Design review of the part built by this model. Coordinates are the model's own, in mm. A direction names the side the tool comes from. Coordinates: 2 decimals unless noted, no trailing zeros. Loops run counter-clockwise (first coordinate to the right, second up) from the corner with the lowest first, then second, coordinate; pieces in that order, holes last. Notation, with made-up numbers: (65, 1.5) -> (114, 1.5) arc R20 cw to (114, 27.5) -> close; hole circle Ø3 at (87.5, -12.75). An arc over 180 degrees is marked (long way). Use a Markdown table: item, result. Add a question column.
Q1. Take a section at B-B on x = -6.5. Write out the cut boundary in (y, z), plus the area to 3 significant figures.
Q2. For faces 4 (the face through (3, 1, -7)), 5 (the face through (-7, 5, -9)), 6 (the face through (-3.9, 5.1, 9.5)), list the 3-axis set-ups (+Z, -Z, +X, -X, +Y, -Y) from which the entire face can be reached by the end or side of a thin tool; tool diameter is ignored.
Q3. Take a section at D-D on y = 5. Count the separate pieces of the cut face and the enclosed holes in it, plus the area to 3 significant figures.
Q4. Take a section at C-C on z = -8. Write out the cut boundary in (x, y).
Q5. Clearance check with flat-ended pins moving along their axes: pin 1 Ø0.5 at (y, z) = (1, 7.5) entering from +X; pin 2 Ø5 at (y, z) = (2, 0.5) entering from +X; pin 3 Ø1.4 at (x, z) = (-13, 8.5) entering from -Y. State where each tip first meets the part, or that it passes through.
Q6. Take a section at A-A on z = 4. Write out the cut boundary in (x, y), plus the area to 3 significant figures.
Q7. For probe 1 along Z at (x, y) = (-4, 7.5); probe 2 along Z at (x, y) = (-11, 7.25); probe 3 along Y at (x, z) = (-3.5, -4.25), list the stretches that pass through material, from the lowest coordinate up.
Q8. Draft analysis for pull direction Y (two halves, no side actions). For faces 1 (the face through (5.15, 5.08, -9.51)), 2 (the face through (-9, 5, 10)), 3 (the face through (-12, 2, -8)), state which applies: pulls with the +Y half, pulls with the -Y half, needs draft (parallel to the pull), parting line crosses it, or undercut.
from build123d import *

# Parameters (mm, degrees)
BASE_DEPTH          = 1.6
SKETCH4_R           = 1.85
ONESIDE_DEPTH       = 1
ANOTHERSIDE_DEPTH   = 1.3
SKETCH5_3_R         = 1.85
PIN_DEPTH           = 1
BOSS_EXTRUDE9_DEPTH = 1.2


with BuildPart() as part:
    # Sketch3 → Base (new body)
    with BuildSketch(Plane(origin=(0, 0, 0), x_dir=(1, 0, 0), z_dir=(0, 1, 0))):
        Polygon((4, 7), (4, 10), (-4, 10), (-4, -10), (4, -10), (4, -7), (2, -7), (2, 7), align=None)
    extrude(amount=BASE_DEPTH)

    # Sketch4 → OneSide (add)
    with BuildSketch(Plane.XY.offset(10)):
        with BuildLine():
            ThreePointArc((-5.064751599, 1.615384615), (-5.175241651, 0.56147099), (-4.276524617, 0))
            Line((-4.276524617, 0), (-4, 0))
            Line((-4, 0), (-4, 1.6))
            Line((-4, 1.6), (4, 1.6))
            Line((4, 1.6), (4, 0))
            Line((4, 0), (7, 0))
            ThreePointArc((7, 0), (12, 5), (7, 10))
            Line((7, 10), (-4.276524617, 10))
            ThreePointArc((-4.276524617, 10), (-5.175241651, 9.43852901), (-5.064751599, 8.384615385))
            ThreePointArc((-5.064751599, 8.384615385), (-3.9, 5), (-5.064751599, 1.615384615))
        make_face()
        with Locations((7, 5)):
            Circle(SKETCH4_R, mode=Mode.SUBTRACT)
    oneside = extrude(amount=-ONESIDE_DEPTH)

    # Sketch5 → AnotherSide (add)
    with BuildSketch(Plane(origin=(0, 0, 9), x_dir=(-1, 0, 0), z_dir=(0, 0, -1))):
        with BuildLine():
            Line((-1, 10), (-1, 0))
            Line((-1, 0), (9.5, 0))
            Line((9.5, 0), (11, 2))
            Line((11, 2), (13.9, 2))
            ThreePointArc((13.9, 2), (14.783156083, 2.530920761), (14.728540367, 3.559929335))
            Line((14.728540367, 3.559929335), (12.160731096, 7.35957601))
            ThreePointArc((12.160731096, 7.35957601), (10.003964328, 9.2989365), (7.189488894, 10))
            Line((7.189488894, 10), (-1, 10))
        make_face()
    anotherside = extrude(amount=ANOTHERSIDE_DEPTH)

    # Sketch5<3> → Pin (add)
    with BuildSketch(Plane(origin=(0, 0, 9), x_dir=(-1, 0, 0), z_dir=(0, 0, -1))):
        with Locations((9.35, 5)):
            Circle(SKETCH5_3_R)
    pin = extrude(amount=-PIN_DEPTH)

    # Mirror1: OneSide, AnotherSide, Pin across plane
    add(oneside.mirror(Plane.XY))
    add(anotherside.mirror(Plane.XY))
    add(pin.mirror(Plane.XY))

    # Sketch6 → Boss-Extrude9 (add)
    with BuildSketch(Plane(origin=(0, 10, 0), x_dir=(1, 0, 0), z_dir=(0, 1, 0))):
        Polygon((-5, 8.547893693), (-5, -8.525702736), (3.4, -9.520454617), (3.4, 9.588680541), align=None)
    extrude(amount=-BOSS_EXTRUDE9_DEPTH)


solid = part.part
Answer list:
| question | item | result |
|---|---|---|
| 1 | outline | (0, -9) -> (10, -9) -> (10, -7.7) -> (0, -7.7) -> close; (0, 7.7) -> (10, 7.7) -> (10, 9) -> (0, 9) -> close |
| 1 | area | 26.0 mm² |
| 2 | face 4 | +X, -Y |
| 2 | face 5 | -Z |
| 2 | face 6 | +Z |
| 3 | separate pieces | 4 |
| 3 | enclosed holes | 0 |
| 3 | area | 70.2 mm² |
| 4 | outline | (-14.73, 3.56) arc R1 ccw to (-13.9, 2) -> (-11, 2) -> (-9.5, 0) -> (4, 0) -> (4, 1.6) -> (1, 1.6) -> (1, 8.8) -> (3.4, 8.8) -> (3.4, 10) -> (-7.19, 10) arc R6 ccw to (-12.16, 7.36) -> close |
| 5 | pin 1 | x = 4 |
| 5 | pin 2 | x = 2 |
| 5 | pin 3 | y = 2 |
| 6 | outline | (-5, 8.8) -> (3.4, 8.8) -> (3.4, 10) -> (-5, 10) -> close; (-4, 0) -> (2, 0) -> (2, 1.6) -> (-4, 1.6) -> close |
| 6 | area | 19.7 mm² |
| 7 | probe 1 | -10 to -7.7, 7.7 to 10 |
| 7 | probe 2 | -9 to -7.7, 7.7 to 9 |
| 7 | probe 3 | 0 to 1.6, 8.8 to 10 |
| 8 | face 1 | undercut |
| 8 | face 2 | needs draft |
| 8 | face 3 | pulls with the -Y half |
